```python
from build123d import *
from build123d.topology import SkipClean

# Parameters (mm, degrees)
SKETCH_1_R          = 2.5
EXTRUDE_1_DEPTH     = 5
SKETCH_2_R          = 10
EXTRUDE_2_DEPTH     = 11.5
CUT_EXTRUDE_START   = -7
CUT_EXTRUDE_1_DEPTH = 7
CUT_EXTRUDE_2_DEPTH = 11.5
SKETCH_5_R          = 3
CUT_EXTRUDE_3_DEPTH = 11.5
SKETCH_6_R          = 1.5
CUT_EXTRUDE_4_DEPTH = 41.165283517


with BuildPart() as part:
    # 草图1 → 凸台-拉伸1 (new body)
    with BuildSketch(Plane(origin=(0, 0, 0), x_dir=(1, 0, 0), z_dir=(0, 1, 0))):
        with BuildLine():
            Line((12, 27.49545417), (12, -27.49545417))
            ThreePointArc((12, -27.49545417), (0, -30), (-12, -27.49545417))
            Line((-12, -27.49545417), (-12, 27.49545417))
            ThreePointArc((-12, 27.49545417), (0, 30), (12, 27.49545417))
        make_face()
        with Locations(Location((0, 22.5, 0), (0, 0, 270))):
            Circle(SKETCH_1_R, mode=Mode.SUBTRACT)
        with Locations(Location((0, -22.5, 0), (0, 0, 270))):
            Circle(SKETCH_1_R, mode=Mode.SUBTRACT)
    extrude(amount=EXTRUDE_1_DEPTH)

    # 草图2 → 凸台-拉伸2 (add)
    with BuildSketch(Plane(origin=(0, 5, 0), x_dir=(1, 0, 0), z_dir=(0, 1, 0))):
        with Locations(Location((0, 0, 0), (0, 0, 270))):
            Circle(SKETCH_2_R)
    extrude(amount=EXTRUDE_2_DEPTH)

    # 草图3 → 切除-拉伸1 (cut)
    with BuildSketch(Plane(origin=(0, 16.5, 0), x_dir=(1, 0, 0), z_dir=(0, 1, 0)).offset(CUT_EXTRUDE_START)):
        with BuildLine():
            Line((9, 4.358898944), (9, -4.358898944))
            ThreePointArc((9, -4.358898944), (10, 0), (9, 4.358898944))
        make_face()
    extrude(amount=CUT_EXTRUDE_1_DEPTH, mode=Mode.SUBTRACT)

    # 草图4 → 切除-拉伸2 (cut)
    with BuildSketch(Plane(origin=(0, 16.5, 0), x_dir=(1, 0, 0), z_dir=(0, 1, 0))):
        with BuildLine():
            Line((2.5, 1.658312395), (2.5, -1.658312395))
            ThreePointArc((2.5, -1.658312395), (-3, 0), (2.5, 1.658312395))
        make_face()
    extrude(amount=-CUT_EXTRUDE_2_DEPTH, mode=Mode.SUBTRACT)

    # 草图5 → 切除-拉伸3 (cut)
    with SkipClean():  # the faces are left unmerged after this step: merging them gives an invalid solid
        with BuildSketch(Plane(origin=(0, 5, 0), x_dir=(1, 0, 0), z_dir=(0, 1, 0))):
            with Locations(Location((0, 0, 0), (0, 0, 270))):
                Circle(SKETCH_5_R)
        extrude(amount=-CUT_EXTRUDE_3_DEPTH, mode=Mode.SUBTRACT)

    # 草图6 → 切除-拉伸4 (cut, through all)
    with SkipClean():  # the faces are left unmerged after this step: merging them gives an invalid solid
        with BuildSketch(Plane(origin=(9, 0, 0), x_dir=(0, 0, -1), z_dir=(1, 0, 0))):
            with Locations((0, 14)):
                Circle(SKETCH_6_R)
        extrude(amount=-CUT_EXTRUDE_4_DEPTH, mode=Mode.SUBTRACT)


solid = part.part
```
Work out the finished part from the listing and answer in its coordinate system (mm). A direction names the side the tool comes from. Coordinates: 2 decimals unless noted, no trailing zeros. Loops run counter-clockwise (first coordinate to the right, second up) from the corner with the lowest first, then second, coordinate; pieces in that order, holes last. Notation, with made-up numbers: (88.5, 65) -> (145.5, 65) arc R15 cw to (145.5, 88) -> close; hole circle Ø1 at (-1.5, -27). An arc over 180 degrees is marked (long way). Answer as CSV lines item,"result".
Q1. The part is cut by section C-C on x = 0. Write down the section's boundary in (y, z).
Findings:
outline,"(0, -30) -> (5, -30) -> (5, -25) -> (0, -25) -> close; (0, -20) -> (5, -20) -> (5, -10) -> (16.5, -10) -> (16.5, -3) -> (0, -3) -> close; (0, 3) -> (16.5, 3) -> (16.5, 10) -> (5, 10) -> (5, 20) -> (0, 20) -> close; (0, 25) -> (5, 25) -> (5, 30) -> (0, 30) -> close"
Q2. For a pull along Z with two mould halves and no side action, classify faces 1 (the face through (2.5, 10, 0)), 2 (the face through (-9.76, 10.67, -2.17)), 3 (the face through (8.2, 5, 6.2)) as +Z half, -Z half, draft (parallel to the pull), parting line (faces both ways), or undercut.
Findings:
face 1,"undercut"
face 2,"parting line"
face 3,"draft"
Q3. Each of these flat-tipped pins is pushed along its axis until it touches: pin 1 (1 mm diameter, centred on x = -6.5, z = 19.5, fed in from +Y); pin 2 (8 mm diameter, centred on x = -8.5, z = -15.5, fed in from -Y); pin 3 (1 mm diameter, centred on y = 13, z = -0.5, fed in from -X); pin 4 (7.5 mm diameter, centred on y = 13, z = -1, fed in from +X). Where does it stop, or does it pass through?
Findings:
pin 1,"stops at y = 5"
pin 2,"stops at y = 0"
pin 3,"stops at x = -9.99"
pin 4,"stops at x = 10"
Q4. The part is cut by section B-B on y = 3.75. Write down the section's boundary in (x, z).
Findings:
outline,"(-12, -27.5) arc R30 ccw to (12, -27.5) -> (12, 27.5) arc R30 ccw to (-12, 27.5) -> close; hole circle Ø6 at (0, 0); hole circle Ø5 at (0, -22.5); hole circle Ø5 at (0, 22.5)"
Q5. The part is cut by section A-A on z = 22.5. Write down the section's boundary in (x, y).
Findings:
outline,"(-12, 0) -> (-2.5, 0) -> (-2.5, 5) -> (-12, 5) -> close; (2.5, 0) -> (12, 0) -> (12, 5) -> (2.5, 5) -> close"
Q6. A tool of negligible diameter and unlimited length cuts with its end or side. For faces 4 (the face through (12, 2, 0)), 5 (the face through (9, 12, 0)), from which of +Z, -Z, +X, -X, +Y, -Y can it reach the whole face along a straight path? Write none if from no direction.
Findings:
face 4,"+Z, -Z, +X, +Y, -Y"
face 5,"+Z, -Z, +X, +Y"
Q7. The part is cut by section D-D on z = 0. Write down the section's boundary in (x, y).
Findings:
outline,"(-12, 0) -> (-3, 0) -> (-3, 12.5) -> (-10, 12.5) -> (-10, 5) -> (-12, 5) -> close; (-10, 15.5) -> (-3, 15.5) -> (-3, 16.5) -> (-10, 16.5) -> close; (2.5, 5) -> (3, 5) -> (3, 0) -> (12, 0) -> (12, 5) -> (10, 5) -> (10, 9.5) -> (9, 9.5) -> (9, 12.5) -> (2.5, 12.5) -> close; (2.5, 15.5) -> (9, 15.5) -> (9, 16.5) -> (2.5, 16.5) -> close"
Q8. Find the intervals of material crossed by probe 1 along X at (y, z) = (2.75, 2.5); probe 2 along Y at (x, z) = (-7.5, 0); probe 3 along X at (y, z) = (9.75, 0), in increasing order.
Findings:
probe 1,"x = -12 to -1.66, 1.66 to 12"
probe 2,"y = 0 to 12.5, 15.5 to 16.5"
probe 3,"x = -10 to -3, 2.5 to 9"
